```python
from build123d import *

# Parameters (mm, degrees)
SKETCH1_W                    = 32
SKETCH1_H                    = 39
BOSS_EXTRUDE1_DEPTH          = 2
SKETCH2_W                    = 5.3
SKETCH2_H                    = 32.65
SKETCH2_W_2                  = 8.89
BOSS_EXTRUDE2_DEPTH          = 3.175
SKETCH10_W                   = 8
SKETCH10_H                   = 5
SKETCH10_W_2                 = 5
SKETCH10_H_2                 = 8
BOSS_EXTRUDE3_DEPTH          = 2
F_52_0_0635_DIAMETER_HOLE1_D = 1.6129
CHAMFER1_SIZE                = 2
CHAMFER3_SIZE                = 1.5
CHAMFER2_SIZE                = 0.75


with BuildPart() as part:
    # Sketch1 → Boss-Extrude1 (new body)
    with BuildSketch(Plane.XY):
        with Locations((0, 157.8)):
            Rectangle(SKETCH1_W, SKETCH1_H)
    extrude(amount=BOSS_EXTRUDE1_DEPTH)

    # Sketch2 → Boss-Extrude2 (add)
    with BuildSketch(Plane.XY.offset(2)):
        with Locations((7, 160.975)):
            Rectangle(SKETCH2_W, SKETCH2_H)
        with Locations((-6.068, 160.975)):
            Rectangle(SKETCH2_W_2, SKETCH2_H)
    extrude(amount=BOSS_EXTRUDE2_DEPTH)

    # Sketch10 → Boss-Extrude3 (add)
    with BuildSketch(Plane.XY.offset(2)):
        with Locations((7, 179.8)):
            Rectangle(SKETCH10_W, SKETCH10_H)
        with Locations((-18.5, 142.3)):
            Rectangle(SKETCH10_W_2, SKETCH10_H_2)
    extrude(amount=-BOSS_EXTRUDE3_DEPTH)

    # #52 (0.0635) Diameter Hole1 (through all)
    with Locations(Plane.XY.offset(5.175)):
        with Locations((7, 174.3), (7, 159.3), (-18.5, 142.3), (7, 179.8)):
            Hole(F_52_0_0635_DIAMETER_HOLE1_D / 2)

    # Chamfer1
    chamfer1_edges = [part.edges().sort_by_distance(p)[0] for p in [
        (16, 177.3, 1),
        (16, 138.3, 1),
        (-16, 177.3, 1),
    ]]
    chamfer(chamfer1_edges, length=CHAMFER1_SIZE)

    # Chamfer3
    chamfer3_edges = [part.edges().sort_by_distance(p)[0] for p in [
        (11, 182.3, 1),
        (3, 182.3, 1),
        (-21, 146.3, 1),
        (-21, 138.3, 1),
        (-16, 146.3, 1),
    ]]
    chamfer(chamfer3_edges, length=CHAMFER3_SIZE)

    # Chamfer2
    chamfer2_edges = [part.edges().sort_by_distance(p)[0] for p in [
        (-21, 142.3, 2),
        (7, 182.3, 2),
        (3, 179.05, 2),
        (-18.5, 146.3, 2),
        (-2.75, 138.3, 2),
        (3.75, 181.55, 2),
        (10.25, 181.55, 2),
        (-20.25, 145.55, 2),
        (-20.25, 139.05, 2),
        (-16.75, 147.05, 2),
        (9.65, 160.975, 2),
        (9.65, 144.65, 3.5875),
        (9.65, 177.3, 3.5875),
        (4.35, 160.975, 2),
        (4.35, 177.3, 3.5875),
        (7, 144.65, 2),
        (4.35, 144.65, 3.5875),
        (9.65, 160.975, 5.175),
        (7, 177.3, 5.175),
        (4.35, 160.975, 5.175),
        (7, 144.65, 5.175),
        (-12.2565, 177.3, 2),
        (-1.623, 160.975, 2),
        (-1.623, 144.65, 3.5875),
        (-1.623, 177.3, 3.5875),
        (-10.513, 160.975, 2),
        (-10.513, 177.3, 3.5875),
        (-6.068, 144.65, 2),
        (-10.513, 144.65, 3.5875),
        (-1.623, 160.975, 5.175),
        (-6.068, 177.3, 5.175),
        (-10.513, 160.975, 5.175),
        (-6.068, 144.65, 5.175),
        (0.6885, 177.3, 2),
        (7, 177.3, 2),
        (11, 179.05, 2),
        (11, 177.3, 1),
        (3, 177.3, 1),
        (12.5, 177.3, 2),
        (16, 157.8, 2),
        (-16, 161.55, 2),
        (-15, 176.3, 2),
        (15, 139.3, 2),
        (15, 176.3, 2),
    ]]
    chamfer(chamfer2_edges, length=CHAMFER2_SIZE)


solid = part.part
```
The listing builds one solid part. Answer for the finished solid, in the listing's coordinates (mm). A direction names the side the tool comes from. Give positions to 0.01 mm unless a question says otherwise; leave off trailing zeros. Order: outer loops, then holes, each group sorted by start corner. A loop starts at its lowest first (then second) coordinate and runs counter-clockwise, first axis right, second up. Notation, with made-up numbers: (72.5, -10) -> (103.5, -10) arc R26 ccw to (103.5, 11) -> close; hole circle Ø7 at (69, 40.5). An arc over 180 degrees is marked (long way). Answer as CSV lines item,"result". Start each with the question number.
Q1. Which of the six approach directions +Z, -Z, +X, -X, +Y, -Y give full straight-line access (tool end or side, diameter ignored) to faces 4 (the flat face through (4.5, 144.8, 2.3)), 5 (the flat face through (16, 158, 1)), 6 (the flat face through (-1.485, 177.003, 2.159)), 7 (the flat face through (-10.65, 177, 2.16)), 8 (the flat face through (-19, 146.3, 1))?
Q2. A cutting plane is placed at A-A (z = 3.6). Determine the outline of the cut face in (x, y), then the cut area to 3 significant figures.
Q3. Determine the mould class of faces 1 (the flat face through (7, 177.3, 4)), 2 (the cylindrical face through (7.17, 158.51, 2.55)), 3 (the flat face through (-10.375, 144.809, 2.297)) for opening direction X: pulls with the +X half, pulls with the -X half, needs draft (parallel to the pull), parting line crosses it, or undercut.
Q4. A cutting plane is placed at D-D (x = 7). Determine the outline of the cut face in (y, z) (3 decimals), then the cut area to 3 significant figures.
Q5. A cutting plane is placed at B-B (x = -18.5). Determine the outline of the cut face in (y, z), then the cut area to 3 significant figures.
Q6. Given pin 1 (2 mm diameter, centred on x = -5.5, z = 0.5, fed in from +Y); pin 2 (1.8 mm diameter, centred on y = 157, z = 3.5, fed in from -X); pin 3 (0.5 mm diameter, centred on y = 158, z = 3.5, fed in from +X), each flat-ended and moving along its own axis, determine where each tip first touches the part or whether it passes through.
Q7. Find the intervals of material crossed by L1, parallel to Y at x = 7, z = 3.6; L2, parallel to X at y = 174.3, z = 4; L3, parallel to Y at x = 7, z = 1.1, in increasing order.
Q8. A cutting plane is placed at C-C (y = 174.3). Determine the outline of the cut face in (x, z) (3 decimals).
Results found:
1,face 4,"+Z, -Y"
1,face 5,"+Z, -Z, +X, +Y, -Y"
1,face 6,"+Z, +Y"
1,face 7,"+Z, -X, +Y"
1,face 8,"+Z, -Z, -X, +Y"
2,outline,"(-10.51, 145.4) -> (-9.76, 144.65) -> (-2.37, 144.65) -> (-1.62, 145.4) -> (-1.62, 176.55) -> (-2.37, 177.3) -> (-9.76, 177.3) -> (-10.51, 176.55) -> close; (4.35, 145.4) -> (5.1, 144.65) -> (8.9, 144.65) -> (9.65, 145.4) -> (9.65, 176.55) -> (8.9, 177.3) -> (5.1, 177.3) -> (4.35, 176.55) -> close; hole circle Ø1.61 at (7, 159.3); hole circle Ø1.61 at (7, 174.3)"
2,area,"457 mm2"
3,face 1,"needs draft"
3,face 2,"undercut"
3,face 3,"pulls with the -X half"
4,outline,"(138.3, 0) -> (158.494, 0) -> (158.494, 5.175) -> (145.4, 5.175) -> (144.65, 4.425) -> (144.65, 2.75) -> (143.9, 2) -> (139.05, 2) -> (138.3, 1.25) -> close; (160.106, 0) -> (173.494, 0) -> (173.494, 5.175) -> (160.106, 5.175) -> close; (175.106, 0) -> (178.994, 0) -> (178.994, 2) -> (178.05, 2) -> (177.3, 2.75) -> (177.3, 4.425) -> (176.55, 5.175) -> (175.106, 5.175) -> close; (180.606, 0) -> (182.3, 0) -> (182.3, 1.25) -> (181.55, 2) -> (180.606, 2) -> close"
4,area,"171 mm2"
5,outline,"(138.3, 0) -> (141.49, 0) -> (141.49, 2) -> (139.05, 2) -> (138.3, 1.25) -> close; (143.11, 0) -> (146.3, 0) -> (146.3, 1.25) -> (145.55, 2) -> (143.11, 2) -> close"
5,area,"12.2 mm2"
6,pin 1,"y = 177.3"
6,pin 2,"x = -10.66"
6,pin 3,"x = 9.65"
7,L1,"144.65 to 158.49, 160.11 to 173.49, 175.11 to 177.3"
7,L2,"-10.51 to -1.62, 4.35 to 6.19, 7.81 to 9.65"
7,L3,"138.3 to 158.49, 160.11 to 173.49, 175.11 to 178.99, 180.61 to 182.3"
8,outline,"(-16, 0) -> (6.194, 0) -> (6.194, 5.175) -> (5.1, 5.175) -> (4.35, 4.425) -> (4.35, 2.75) -> (3.6, 2) -> (-0.873, 2) -> (-1.623, 2.75) -> (-1.623, 4.425) -> (-2.373, 5.175) -> (-9.763, 5.175) -> (-10.513, 4.425) -> (-10.513, 2.75) -> (-11.263, 2) -> (-15.25, 2) -> (-16, 1.25) -> close; (7.806, 0) -> (16, 0) -> (16, 1.25) -> (15.25, 2) -> (10.4, 2) -> (9.65, 2.75) -> (9.65, 4.425) -> (8.9, 5.175) -> (7.806, 5.175) -> close"
